Answer from the drawing. Dimensions are ordinates in mm from the lowest x, y and z of the part. Round coordinates to 2 decimals unless told otherwise and drop trailing zeros. Write each loop counter-clockwise with the first axis right and the second up, starting at its lowest first coordinate (ties: lowest second). Pieces come first, ordered by that corner, then holes. Notation, with made-up numbers: (38, 34) - (70, 34) arc R12 ccw to (70, 38) - close; hole circle Ø7 at (87, 55.5). An arc over 180 degrees is marked (long way). Write item = value, one per line. Start each with the question number.
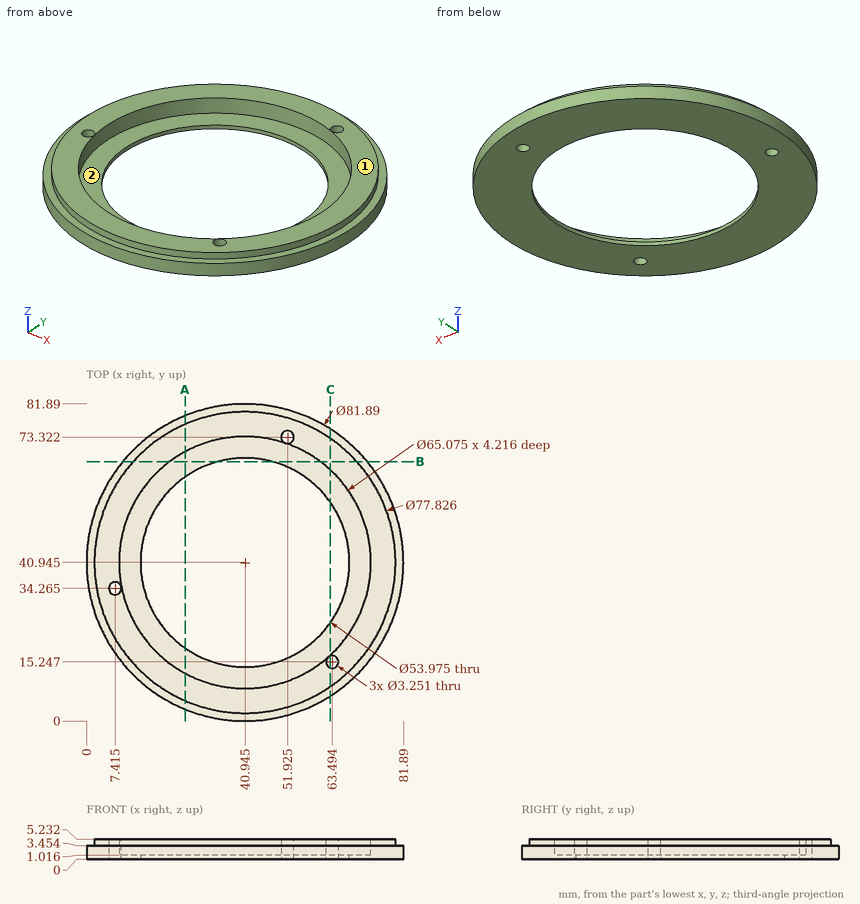
1. Consider line 1 (X direction, y = 41, z = 0.85); line 2 (Y direction, x = 41.5, z = 4.1) (1 decimal); line 3 (X direction, y = 44, z = 0.95) (1 decimal). Determine where each line is inside the solid, lowest interval first.
2. Each of these flat-tipped pins is pushed along its axis until it touches: pin 1 (1.5 mm diameter, centred on y = 29, z = 2.5, fed in from +X); pin 2 (2 mm diameter, centred on x = 35, z = 2, fed in from +Y); pin 3 (10 mm diameter, centred on x = 56.5, y = 23.5, fed in from +Z). Where does it stop, or does it pass through?
3. For a pull along X with two mould halves and no side action, classify the marked faces 1 and 2 as released by +X, released by -X, zero draft, split by the parting line, or undercut.
4. Find section C-C on x = 63. Give the number of separate pieces and of enclosed holes in the cut face, plus the area to 3 significant figures.
5. Find section B-B on y = 67. Give the vertices of the cut face in (x, z) (1 decimal), plus the area to 3 significant figures.
6. Find section A-A on x = 25.5. Give the vertices of the cut face in (y, z) (1 decimal).
Answer key:
q1.line_1 = 0 to 13.96, 67.93 to 81.89
q1.line_2 = 2 to 8.4, 73.5 to 79.9
q1.line_3 = 0.1 to 14.1, 67.8 to 81.8
q2.pin_1 = 80.33
q2.pin_2 = 81.59
q2.pin_3 = 1.02
q3.face_1 = zero draft
q3.face_2 = undercut
q4.separate_pieces = 3
q4.enclosed_holes = 0
q4.area = 103 mm²
q5.outline = (9.4, 0) - (33.9, 0) - (33.9, 1) - (21.5, 1) - (21.5, 5.2) - (12, 5.2) - (12, 3.5) - (9.4, 3.5) - close; (48, 0) - (72.5, 0) - (72.5, 3.5) - (69.8, 3.5) - (69.8, 5.2) - (60.4, 5.2) - (60.4, 1) - (48, 1) - close
q5.area = 142 mm²
q6.outline = (3, 0) - (18.8, 0) - (18.8, 1) - (12.3, 1) - (12.3, 5.2) - (5.2, 5.2) - (5.2, 3.5) - (3, 3.5) - close; (63.1, 0) - (78.9, 0) - (78.9, 3.5) - (76.7, 3.5) - (76.7, 5.2) - (69.6, 5.2) - (69.6, 1) - (63.1, 1) - close
